```python
from build123d import *

# Parameters (mm, degrees)
SKETCH2_R           = 40
SKETCH2_R_2         = 7.5
BOSS_EXTRUDE1_DEPTH = 5


with BuildPart() as part:
    # Sketch2 → Boss-Extrude1 (new, symmetric)
    with BuildSketch(Plane(origin=(0, 0, 0), x_dir=(1, 0, 0), z_dir=(0, 1, 0))):
        with Locations(Location((0, 0, 0), (0, 0, 270))):
            Circle(SKETCH2_R)
        with Locations(Location((0, 0, 0), (0, 0, 270))):
            Circle(SKETCH2_R_2, mode=Mode.SUBTRACT)
        with BuildLine():
            Line((-2, 35.944401511), (-2, 9.287087811))
            ThreePointArc((-2, 9.287087811), (-8.227241336, 4.75), (-9.042853971, -2.911493098))
            Line((-9.042853971, -2.911493098), (-32.128764833, -16.240149948))
            ThreePointArc((-32.128764833, -16.240149948), (-31.176914536, 18), (-2, 35.944401511))
        make_face(mode=Mode.SUBTRACT)
        with BuildLine():
            Line((2, 35.944401511), (2, 9.287087811))
            ThreePointArc((2, 9.287087811), (8.227241336, 4.75), (9.042853971, -2.911493098))
            Line((9.042853971, -2.911493098), (32.128764833, -16.240149948))
            ThreePointArc((32.128764833, -16.240149948), (31.176914536, 18), (2, 35.944401511))
        make_face(mode=Mode.SUBTRACT)
        with BuildLine():
            Line((-7.042853971, -6.375594713), (-30.128764833, -19.704251563))
            ThreePointArc((-30.128764833, -19.704251563), (0, -36), (30.128764833, -19.704251563))
            Line((30.128764833, -19.704251563), (7.042853971, -6.375594713))
            ThreePointArc((7.042853971, -6.375594713), (0, -9.5), (-7.042853971, -6.375594713))
        make_face(mode=Mode.SUBTRACT)
    extrude(amount=BOSS_EXTRUDE1_DEPTH, both=True)


solid = part.part
```
Part model, mm, in its own coordinate system. A direction names the side the tool comes from. Give positions to 0.01 mm unless a question says otherwise; leave off trailing zeros. Order: outer loops, then holes, each group sorted by start corner. A loop starts at its lowest first (then second) coordinate and runs counter-clockwise, first axis right, second up. Notation, with made-up numbers: (-39.5, 13.25) - (-10.5, 13.25) arc R17 cw to (-10.5, 27.25) - close; hole circle Ø2 at (-12.5, -18.75). An arc over 180 degrees is marked (long way). Use one line per item in the form item = value.
Item 1: Probe probe 1 along X at (y, z) = (1.5, 0); probe 2 along Z at (x, y) = (3, -4); probe 3 along Z at (x, y) = (8, 3). List the from-to ranges inside material, lowest first. Write a range as from..to.
Solution:
probe_1 = -40..-36, -9.5..-7.5, 7.5..9.5, 36..40
probe_2 = -39.89..-35.87, -9.01..-6.87, 6.87..9.01, 35.87..39.89
probe_3 = -39.19..-35.1, -5.12..6.93, 35.1..39.19
Item 2: Two-plate mould, pull along Z, no slides. Class faces 1 (the face through (-39.05, 0.07, -8.67)), 2 (the face through (-6, -5, 6)), 3 (the face through (-31.42, 0.07, -17.57)), 4 (the face through (-2, 0, -23)): released by +Z, released by -Z, zero draft, split by the parting line, or undercut.
Solution:
face_1 = split by the parting line
face_2 = zero draft
face_3 = undercut
face_4 = undercut
Item 3: Pin check, flat tips, straight feed: pin 1 Ø5 at (y, z) = (-1, -19) entering from -X; pin 2 Ø6 at (y, z) = (-3.5, -25) entering from +X; pin 3 Ø3 at (x, y) = (-16, -2) entering from -Z. Stop position of each tip, or through.
Solution:
pin_1 = -36.44
pin_2 = 33.41
pin_3 = -37.28
Item 4: Slice it at B-B on x = 34. Give the cut face in (y, z).
Solution:
outline = (-5, -21.07) - (5, -21.07) - (5, -11.83) - (-5, -11.83) - close; (-5, 11.83) - (5, 11.83) - (5, 21.07) - (-5, 21.07) - close
Item 5: Which spindle directions (+Z, -Z, +X, -X, +Y, -Y) get a long thin tool onto all of the face, cutting with end or side? Do faces 5 (the face through (-6, 5, 6)), 6 (the face through (8.2, 0.1, -4.8)). Say none if no direction does.
Solution:
face_5 = +Z, -Z, +X, -X, +Y
face_6 = +Y, -Y
Item 6: Slice it at A-A on z = 0. Give the cut face in (x, y).
Solution:
outline = (-40, -5) - (-36, -5) - (-36, 5) - (-40, 5) - close; (-9.5, -5) - (-7.5, -5) - (-7.5, 5) - (-9.5, 5) - close; (7.5, -5) - (9.5, -5) - (9.5, 5) - (7.5, 5) - close; (36, -5) - (40, -5) - (40, 5) - (36, 5) - close
Item 7: Slice it at C-C on y = 1.5. Give the cut face in (x, z), and give its area (3 significant figures).
Solution:
outline = circle Ø80 at (0, 0); hole (-32.13, 16.24) arc R36 ccw to (-2, -35.94) - (-2, -9.29) arc R9.5 cw to (-9.04, 2.91) - close; hole (-30.13, 19.7) - (-7.04, 6.38) arc R9.5 cw to (7.04, 6.38) - (30.13, 19.7) arc R36 ccw to start; hole circle Ø15 at (0, 0); hole (2, -35.94) arc R36 ccw to (32.13, 16.24) - (9.04, 2.91) arc R9.5 cw to (2, -9.29) - close
area = 1,380 mm2
Item 8: Slice it at D-D on x = 0. Give the cut face in (y, z).
Solution:
outline = (-5, -40) - (5, -40) - (5, -7.5) - (-5, -7.5) - close; (-5, 7.5) - (5, 7.5) - (5, 9.5) - (-5, 9.5) - close; (-5, 36) - (5, 36) - (5, 40) - (-5, 40) - close
